The listing builds one solid part. Answer for the finished solid, in the listing's coordinates (mm). Give positions to 0.01 mm unless a question says otherwise; leave off trailing zeros. Loops run counter-clockwise (first coordinate to the right, second up) from the corner with the lowest first, then second, coordinate; pieces in that order, holes last.
Item 1: Section B-B, the plane z = 2.5 is taken. Give the vertices of the cut face in (x, y).
Item 2: Consider line 1 along X through (y, z) = (-6, 2.1); line 2 along Y through (x, z) = (0, 2.45); line 3 along Y through (x, z) = (-35, 1.25). Determine where each line is inside the solid, lowest interval first.
Item 3: Section A-A, the plane x = 0 is taken. Give the vertices of the cut face in (y, z) (3 decimals), and give its area (3 significant figures).
Item 4: Section C-C, the plane y = -7.62 is taken. Give the vertices of the cut face in (x, z) (3 decimals), and give its area (3 significant figures).
Item 5: Each of these flat-tipped pins is pushed along its axis until it touches: pin 1 Ø1 at (x, z) = (-40, 1) entering from -Y; pin 2 Ø1 at (y, z) = (-11.5, 2) entering from +X. Where does it stop, or does it pass through?
Item 6: Section D-D, the plane x = -35 is taken. Give the vertices of the cut face in (y, z) (3 decimals), and give its area (3 significant figures).
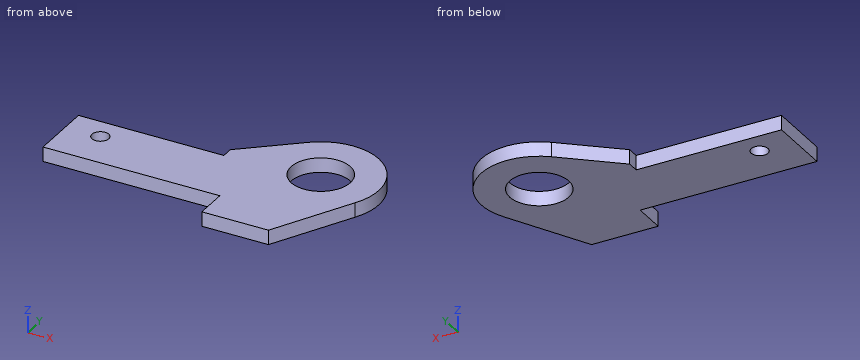
from build123d import *

# Parameters (mm, degrees)
SKETCH1_R                = 6.477
BOSS_EXTRUDE1_DEPTH      = 3.175
CUT_EXTRUDE1_REACH       = 71.794
SKETCH2_W                = 36.544437467
SKETCH2_H                = 39.878
SKETCH3_W                = 3.175
SKETCH3_H                = 13.97
BOSS_EXTRUDE2_DEPTH      = 22.86
M3_CLEARANCE_HOLE1_D     = 3.7
M3_CLEARANCE_HOLE1_DEPTH = 25.4
M3_CLEARANCE_HOLE1_TIP   = 1.111592145
SKETCH7_W                = 3.175
SKETCH7_H                = 7.112
CUT_EXTRUDE2_DEPTH       = 15.875


with BuildPart() as part:
    # Sketch1 → Boss-Extrude1 (new body)
    with BuildSketch(Plane.XY):
        with BuildLine():
            Line((-8.141025641, 9.747497192), (-19.812, 0))
            Line((-19.812, 0), (-19.812, -2.54))
            Line((-19.812, -2.54), (-28.7909, -2.54))
            Line((-28.7909, -2.54), (-28.7909, -63.5))
            Line((-28.7909, -63.5), (-19.812, -63.5))
            Line((-19.812, -63.5), (10.998522628, -6.35))
            ThreePointArc((10.998522628, -6.35), (8.174574987, 9.719378775), (-8.141025641, 9.747497192))
        make_face()
        Circle(SKETCH1_R, mode=Mode.SUBTRACT)
    extrude(amount=BOSS_EXTRUDE1_DEPTH)

    # Sketch2 → Cut-Extrude1 (cut, up to next)
    with BuildSketch(Plane.XY.offset(3.175), mode=Mode.PRIVATE) as cut_extrude1_sk1:
        with Locations((-10.518681266, -43.561)):
            Rectangle(SKETCH2_W, SKETCH2_H)
    cut_extrude1_tool1 = extrude(cut_extrude1_sk1.sketch, amount=-CUT_EXTRUDE1_REACH, mode=Mode.PRIVATE) & part.part
    add(cut_extrude1_tool1.solids().sort_by_distance((-10.518681, -43.561, 3.175))[0], mode=Mode.SUBTRACT)

    # Sketch3 → Boss-Extrude2 (add)
    with BuildSketch(Plane.ZY.offset(28.7909)):
        with Locations((1.5875, -9.525)):
            Rectangle(SKETCH3_W, SKETCH3_H)
    extrude(amount=BOSS_EXTRUDE2_DEPTH)

    # M3 Clearance Hole1
    with Locations(Plane(origin=(0, 0, 0), x_dir=(-1, 0, 0), z_dir=(0, 0, -1))):
        with Locations((44.0309, -7.62)):
            Hole(M3_CLEARANCE_HOLE1_D / 2, depth=M3_CLEARANCE_HOLE1_DEPTH)
            with Locations((0, 0, -(M3_CLEARANCE_HOLE1_DEPTH + M3_CLEARANCE_HOLE1_TIP / 2))):  # 118° drill point
                Cone(0, M3_CLEARANCE_HOLE1_D / 2, M3_CLEARANCE_HOLE1_TIP, mode=Mode.SUBTRACT)

    # Sketch7 → Cut-Extrude2 (cut)
    with BuildSketch(Plane.ZY.offset(28.7909)):
        with Locations((1.5875, -20.066)):
            Rectangle(SKETCH7_W, SKETCH7_H)
    extrude(amount=-CUT_EXTRUDE2_DEPTH, mode=Mode.SUBTRACT)


solid = part.part
Worked answers:
1. outline: (-51.65, -16.51) - (-12.92, -16.51) - (-12.92, -23.62) - (1.69, -23.62) - (11, -6.35) arc R12.7 ccw to (-8.14, 9.75) - (-19.81, 0) - (-19.81, -2.54) - (-51.65, -2.54) - close; hole circle Ø3.7 at (-44.03, -7.62); hole circle Ø12.95 at (0, 0)
2. line 1: x = -51.65 to -44.92, -43.14 to -2.44, 2.44 to 11.19
2. line 2: y = -23.62 to -6.48, 6.48 to 12.7
2. line 3: y = -16.51 to -2.54
3. outline: (-23.622, 0) - (-6.477, 0) - (-6.477, 3.175) - (-23.622, 3.175) - close; (6.477, 0) - (12.7, 0) - (12.7, 3.175) - (6.477, 3.175) - close
3. area: 74.2 mm2
4. outline: (-51.651, 0) - (-45.881, 0) - (-45.881, 3.175) - (-51.651, 3.175) - close; (-42.181, 0) - (10.314, 0) - (10.314, 3.175) - (-42.181, 3.175) - close
4. area: 185 mm2
5. pin 1: stops at y = -16.51
5. pin 2: stops at x = 8.49
6. outline: (-16.51, 0) - (-2.54, 0) - (-2.54, 3.175) - (-16.51, 3.175) - close
6. area: 44.4 mm2
